```python
from build123d import *

# Parameters (mm, degrees)
BOSS_EXTRUDE1_DEPTH = 444.5
SKETCH3_R           = 1.651
SKETCH3_R_2         = 4.826
SKETCH3_R_3         = 1.5875
SKETCH3_R_4         = 3.175
CUT_EXTRUDE1_DEPTH  = 446.700343561
SKETCH4_R           = 3.175
CUT_EXTRUDE2_DEPTH  = 447.547694121
LPATTERN1_COUNT     = 35
LPATTERN1_PITCH     = 25.4
CUT_EXTRUDE3_START  = -12.7
CUT_EXTRUDE3_DEPTH  = 459.400343561


with BuildPart() as part:
    # Sketch2 → Boss-Extrude1 (new, symmetric)
    with BuildSketch(Plane(origin=(0, 0, 0), x_dir=(1, 0, 0), z_dir=(0, 1, 0))):
        with BuildLine():
            Line((-12.7, 0), (-12.7, 22.225))
            ThreePointArc((-12.7, 22.225), (-11.77006403, 24.47006403), (-9.525, 25.4))
            Line((-9.525, 25.4), (9.525, 25.4))
            ThreePointArc((9.525, 25.4), (11.77006403, 24.47006403), (12.7, 22.225))
            Line((12.7, 22.225), (12.7, 0))
            Line((12.7, 0), (15.875, 0))
            Line((15.875, 0), (15.875, 22.225))
            ThreePointArc((15.875, 22.225), (14.015128061, 26.715128061), (9.525, 28.575))
            Line((9.525, 28.575), (-9.525, 28.575))
            ThreePointArc((-9.525, 28.575), (-14.015128061, 26.715128061), (-15.875, 22.225))
            Line((-15.875, 22.225), (-15.875, 0))
            Line((-15.875, 0), (-12.7, 0))
        make_face()
    extrude(amount=BOSS_EXTRUDE1_DEPTH, both=True)

    # Sketch3 → Cut-Extrude1 (cut, through all)
    with BuildSketch(Plane(origin=(0, 0, -28.575), x_dir=(-1, 0, 0), z_dir=(0, 0, -1))):
        with Locations((0, 444.5)):
            Circle(SKETCH3_R)
        with Locations((-2.032, 361.95)):
            Circle(SKETCH3_R_2)
        with Locations((-2.032, 336.55)):
            Circle(SKETCH3_R_2)
        with Locations((-2.032, 107.95)):
            Circle(SKETCH3_R_2)
        with Locations((-2.032, 82.55)):
            Circle(SKETCH3_R_2)
        with Locations((-2.032, -107.95)):
            Circle(SKETCH3_R_2)
        with Locations((-2.032, -82.55)):
            Circle(SKETCH3_R_2)
        with Locations((0, -241.3)):
            Circle(SKETCH3_R_3)
        with Locations((0, 118.11)):
            Circle(SKETCH3_R_4)
        with Locations((-2.032, -336.55)):
            Circle(SKETCH3_R_2)
        with Locations((-2.032, -361.95)):
            Circle(SKETCH3_R_2)
        with Locations((0, 159.512)):
            Circle(SKETCH3_R_4)
        with Locations((0, -159.512)):
            Circle(SKETCH3_R_4)
        with Locations((0, -118.11)):
            Circle(SKETCH3_R_4)
    extrude(amount=-CUT_EXTRUDE1_DEPTH, mode=Mode.SUBTRACT)

    # Sketch4 → Cut-Extrude2 (cut, through all)
    with BuildSketch(Plane(origin=(15.875, 0, 0), x_dir=(0, 0, -1), z_dir=(1, 0, 0))):
        with Locations((12.7, 431.8)):
            Circle(SKETCH4_R)
    cut_extrude2 = extrude(amount=-CUT_EXTRUDE2_DEPTH, mode=Mode.SUBTRACT)

    # LPattern1: Cut-Extrude2 ×35
    with Locations(*[(0, -i * LPATTERN1_PITCH, 0) for i in range(1, LPATTERN1_COUNT)]):
        add(cut_extrude2, mode=Mode.SUBTRACT)

    # Sketch5 → Cut-Extrude3 (cut, through all)
    with BuildSketch(Plane(origin=(0, 0, 0), x_dir=(0, 0, -1), z_dir=(1, 0, 0)).offset(CUT_EXTRUDE3_START)):
        Polygon((0, 100.838), (0, -100.838), (28.575, -76.835), (28.575, 76.835), align=None)
    extrude(amount=CUT_EXTRUDE3_DEPTH, mode=Mode.SUBTRACT)


solid = part.part
```
The model under review builds one solid part; all positions refer to its coordinate system, in mm. A direction names the side the tool comes from. Round coordinates to 2 decimals unless told otherwise and drop trailing zeros.
(1) For P1, Ø4, axis at y = -381, z = -12.7, coming from the -X side; P2, Ø5, axis at y = -137.5, z = -25.5, coming from the -X side; P3, Ø3, axis at x = -8, y = -148, coming from the +Z side, all flat-tipped, find the tip position at first contact; note any pin that passes through.
Working result:
P1: passes through
P2: stops at x = -15.83
P3: stops at z = -25.4
(2) Tool access review of faces 5 (the face through (13.16, -84.45, -19.51)), 6 (the face through (0, 263, -28.575)), 7 (the face through (0, -259, -25.4)): name each direction out of +Z, -Z, +X, -X, +Y, -Y from which nothing blocks a thin tool from reaching the whole face with its end or side.
Working result:
face 5: +Z, +X
face 6: -Z, +X, -X, +Y, -Y
face 7: +Z, +Y, -Y
(3) Wall thickness on L1, parallel to X at y = -273, z = -2.25 (3 decimals); L2, parallel to Z at x = 2.5, y = 394.5 (3 decimals); L3, parallel to X at y = -81, z = -5 (3 decimals): over which ranges is each line inside the solid? List them lowest first.
Working result:
L1: x = -15.875 to -12.7, 12.7 to 15.875
L2: z = -28.575 to -25.4
L3: x = -15.875 to -12.7
(4) Mouldability with a two-part tool opening along X and no side actions: class faces 1 (the face through (-15.875, 6, -11)), 2 (the face through (12.7, -261, -11)), 3 (the face through (0, 265, -25.4)), 4 (the face through (13.162, 84.335, -19.646)) as released by +X, released by -X, zero draft, split by the parting line, or undercut.
Working result:
face 1: released by -X
face 2: undercut
face 3: undercut
face 4: zero draft
